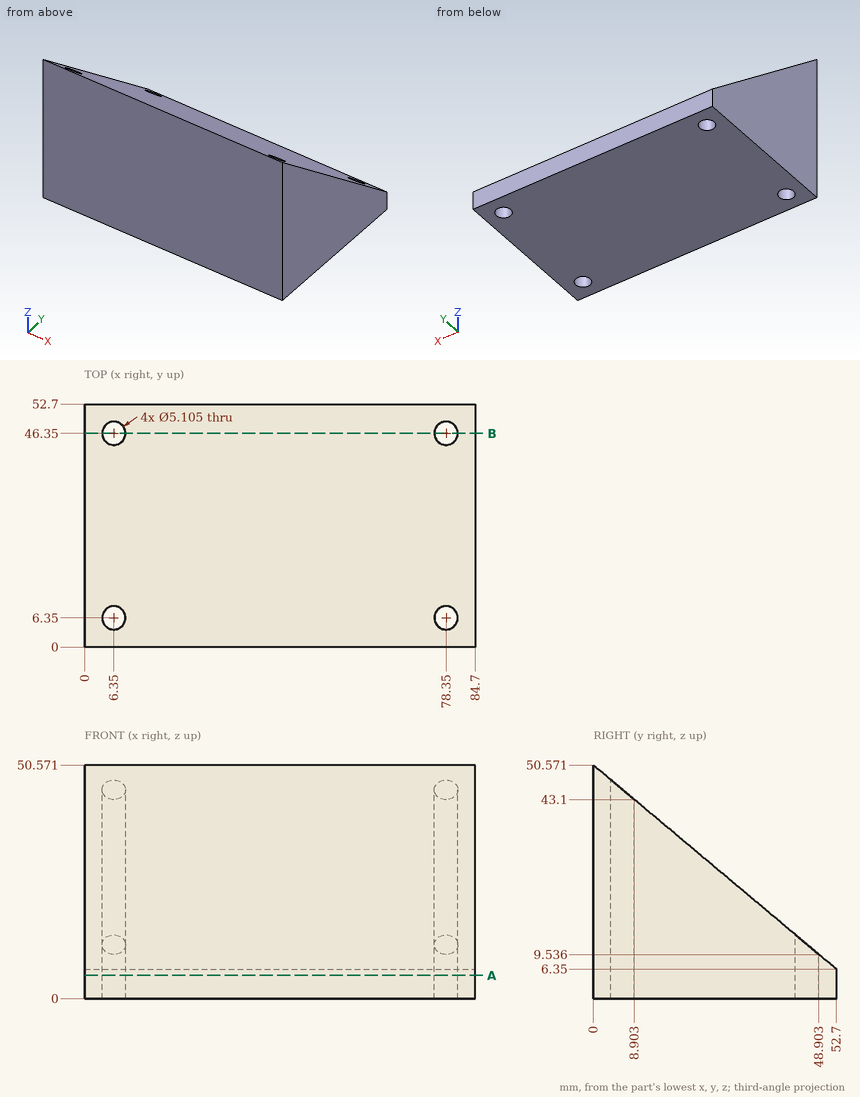
Could you check a few things on this drawing? It's one solid part, dimensions in mm from its lowest x, y, z. Round coordinates to 2 decimals unless told otherwise and drop trailing zeros. Loops run counter-clockwise (first coordinate to the right, second up) from the corner with the lowest first, then second, coordinate; pieces in that order, holes last. Notation, with made-up numbers: M 15,41 L 22,41 A20 ccw 22,56 Z; hole C 61.5,83.25 d2. An arc over 180 degrees is marked long. Write item = value, one per line. Start each with the question number.
(1) Suppose I cut it at B-B on y = 46.35. Write out the boundary of the cut face in (x, z).
(2) Suppose I cut it at A-A on z = 5. Give the number of separate pieces and of enclosed holes in the cut face, plus the area to 3 significant figures.
(3) I need wall thicknesses on line 1 along X through (y, z) = (46.35, 8); line 2 along Y through (x, z) = (78, 4); line 3 along Y through (x, z) = (79.5, 8) (1 decimal). Which ranges of each line are inside material? Lowest first, please.
(4) I'm going to push flat-ended pins straight in: P1, Ø6, axis at x = 6.35, y = 6.35, coming from the +Z side; P2, Ø8, axis at x = 55, y = 10.5, coming from the +Z side; P3, Ø8, axis at x = 35.5, z = 11, coming from the +Y side (1 decimal). Where does each tip first touch, or does it pass through?
Answer block:
q1.outline = M 0,0 L 3.8,0 L 3.8,11.68 L 0,11.68 Z; M 8.9,0 L 75.8,0 L 75.8,11.68 L 8.9,11.68 Z; M 80.9,0 L 84.7,0 L 84.7,11.68 L 80.9,11.68 Z
q2.separate_pieces = 1
q2.enclosed_holes = 4
q2.area = 4,380 mm²
q3.line_1 = 0 to 3.8, 8.9 to 75.8, 80.9 to 84.7
q3.line_2 = 0 to 3.82, 8.88 to 43.82, 48.88 to 52.7
q3.line_3 = 0 to 4.1, 8.6 to 44.1, 48.6 to 50.7
q4.P1 = 47.76
q4.P2 = 45.12
q4.P3 = 51.9
